Input: part model. Units: mm. Frame: model coordinates. Face numbers are marked on the shaded views. A direction names the side the tool comes from. Coordinates: 2 decimals unless noted, no trailing zeros. Write each loop counter-clockwise with the first axis right and the second up, starting at its lowest first coordinate (ties: lowest second). Pieces come first, ordered by that corner, then holes. Notation, with made-up numbers: (79, 21) -> (107, 21) arc R22 cw to (107, 47) -> close; hole circle Ø9 at (29.5, -38). An arc over 180 degrees is marked (long way). One line per question, with ' | ' between items. Start each with the question number.
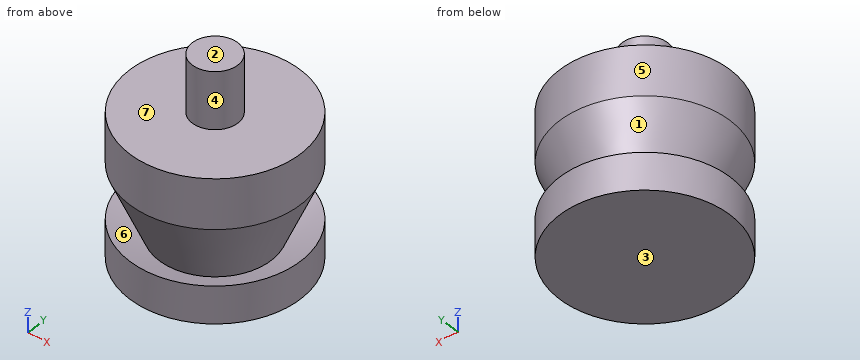
```python
from build123d import *

# Parameters (mm, degrees)
F2_R     = 4
F3_DEPTH = 10


with BuildPart() as f1:
    # F0 (on Front) → F1 (revolve)
    with BuildSketch(Plane.XZ):
        Polygon((0, 0), (0, 25), (-15, 25), (-15, 16.248118), (-9.843752, 4.150979), (-15, 6.522967), (-15, 0), align=None)
    revolve(axis=Axis((0, 0, 12.5), (0, 0, -1)))

    # F2 (on face) → F3 (join)
    with BuildSketch(Plane.XY.offset(25)):
        Circle(F2_R)
    extrude(amount=F3_DEPTH)


solid = f1.part
```
1) Section A-A, the plane x = 0. Return loops of the section in (y, z).
2) First-contact query: P1, Ø5, axis at y = -3.5, z = 27, coming from the +X side; P2, Ø3, axis at x = 11.5, y = -3.5, coming from the +Z side; P3, Ø12, axis at x = -8, z = 24, coming from the +Y side. Flat tips, straight axial feed; report the tip coordinate or a pass-through.
3) Access query for the marked faces 5, 6 and 7. Directions: +Z, -Z, +X, -X, +Y, -Y. A direction counts if a zero-diameter tool reaches every point of the face in a straight line with its end or side. Return the directions, or none.
4) Section C-C, the plane z = 28. Return loops of the section in (x, y), then the cut area to 3 significant figures.
5) Ray query, line 1 (Z direction, x = 4.75, y = -2); line 2 (Z direction, x = 5.75, y = 9.75); line 3 (Z direction, x = 7.5, y = 7.5). Return the intervals inside material, ascending.
6) Section D-D, the plane z = 2.5. Return loops of the section in (x, y), then the cut area to 3 significant figures.
7) Pull-direction query (Z, two-part tool) for the marked faces 1, 2, 3 and 4; classes: released by +Z, released by -Z, zero draft, split by the parting line, or undercut.
Answer block:
1) outline: (-15, 0) -> (15, 0) -> (15, 6.52) -> (9.84, 4.15) -> (15, 16.25) -> (15, 25) -> (4, 25) -> (4, 35) -> (-4, 35) -> (-4, 25) -> (-15, 25) -> (-15, 16.25) -> (-9.84, 4.15) -> (-15, 6.52) -> close
2) P1: stops at x = 14.87 | P2: stops at z = 25 | P3: stops at y = 14.87
3) face 5: +Z, -Z | face 6: none | face 7: +Z
4) outline: circle Ø8 at (0, 0) | area: 50.3 mm2
5) line 1: z = 0 to 25 | line 2: z = 0 to 4.83, 7.61 to 25 | line 3: z = 0 to 4.5, 5.94 to 25
6) outline: circle Ø30 at (0, 0) | area: 707 mm2
7) face 1: undercut | face 2: released by +Z | face 3: released by -Z | face 4: zero draft
